Verification items for the finished model (mm, model axes). Face numbers are marked on the shaded views. A direction names the side the tool comes from. Round coordinates to 2 decimals unless told otherwise and drop trailing zeros. Loops run counter-clockwise (first coordinate to the right, second up) from the corner with the lowest first, then second, coordinate; pieces in that order, holes last. Notation, with made-up numbers: (-17.5, 66) -> (-10.5, 66) arc R10 ccw to (-10.5, 80) -> close; hole circle Ø10 at (5, -34.75). An arc over 180 degrees is marked (long way). Use a Markdown table: item, result. Add a question column.
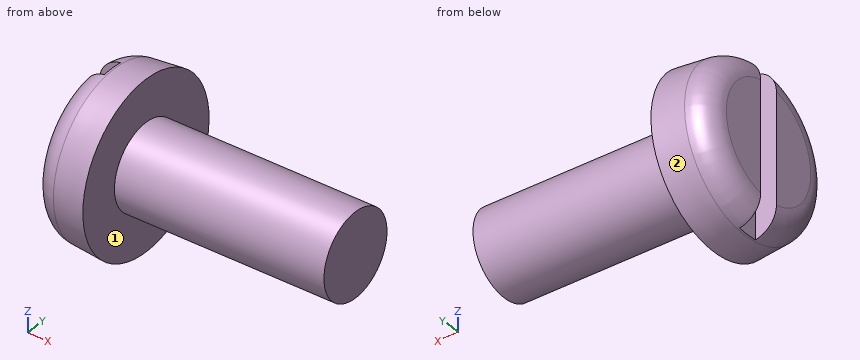
```python
from build123d import *

# Parameters (mm, degrees)
FILLET2_R  = 0.6
SKETCH2_W  = 4
SKETCH2_H  = 0.5
SLOT_DEPTH = 0.5


with BuildPart() as part:
    # BodySke → Base-Revolve (revolve)
    with BuildSketch(Plane.XY, mode=Mode.PRIVATE) as base_revolve_sk:
        Polygon((1.3, 1), (1.3, 2), (0, 1.886264737), (0, 0), (6.3, 0), (6.3, 1), align=None)
    revolve(base_revolve_sk.sketch.rotate(Axis((-25.4, 0, 0), (1, 0, 0)), 90), axis=Axis((-25.4, 0, 0), (1, 0, 0)))  # turned: the seam where the file's is

    # Fillet2
    fillet2_edges = [part.edges().sort_by_distance(p)[0] for p in [
        (0, 0, -1.886264737),
    ]]
    fillet(fillet2_edges, radius=FILLET2_R)

    # Sketch2 → Slot (cut)
    with BuildSketch(Plane(origin=(0, 0, 0), x_dir=(0, 0, -1), z_dir=(1, 0, 0))):
        Rectangle(SKETCH2_W, SKETCH2_H)
    extrude(amount=SLOT_DEPTH, mode=Mode.SUBTRACT)


solid = part.part
```
1) Thickness scan on line 1 (X direction, y = 0.2, z = 1.3); line 2 (X direction, y = -1.35, z = 0.05); line 3 (Z direction, x = 4.5, y = -0.3). Record the ranges inside material, lowest first.
2) Sectioned sample at C-C on x = 2.75. Enter the section's corners in (y, z), then the cut area to 3 significant figures.
3) Go/stop test with flat-tipped pins: pin 1 (0.6 mm diameter, centred on x = 0.5, z = 0, fed in from +Y); pin 2 (1.5 mm diameter, centred on x = 1.5, z = 1, fed in from -Y). Record where each tip stops, or that it passes through.
4) Sectioned sample at A-A on z = 0. Enter the section's corners in (x, y), then the cut area to 3 significant figures.
5) Sectioned sample at B-B on y = 0. Enter the section's corners in (x, z), then the cut area to 3 significant figures.
6) Access from +Z, -Z, +X, -X, +Y, -Y to the whole of each face (thin tool, end or side, straight path). Record for the marked faces 1 and 2.
Geometry results:
| question | item | result |
|---|---|---|
| 1 | line 1 | 0.5 to 1.3 |
| 1 | line 2 | 0 to 1.3 |
| 1 | line 3 | -0.95 to 0.95 |
| 2 | outline | circle Ø2 at (0, 0) |
| 2 | area | 3.14 mm^2 |
| 3 | pin 1 | y = 1.96 |
| 3 | pin 2 | y = -1.98 |
| 4 | outline | (0, -1.34) arc R0.6 ccw to (0.55, -1.93) -> (1.3, -2) -> (1.3, -1) -> (6.3, -1) -> (6.3, 1) -> (1.3, 1) -> (1.3, 2) -> (0.55, 1.93) arc R0.6 ccw to (0, 1.34) -> (0, 0.25) -> (0.5, 0.25) -> (0.5, -0.25) -> (0, -0.25) -> close |
| 4 | area | 14.7 mm^2 |
| 5 | outline | (0.5, -1.93) arc R0.6 ccw to (0.55, -1.93) -> (1.3, -2) -> (1.3, -1) -> (6.3, -1) -> (6.3, 1) -> (1.3, 1) -> (1.3, 2) -> (0.55, 1.93) arc R0.6 ccw to (0.5, 1.93) -> close |
| 5 | area | 13.1 mm^2 |
| 6 | face 1 | +X |
| 6 | face 2 | -X |
